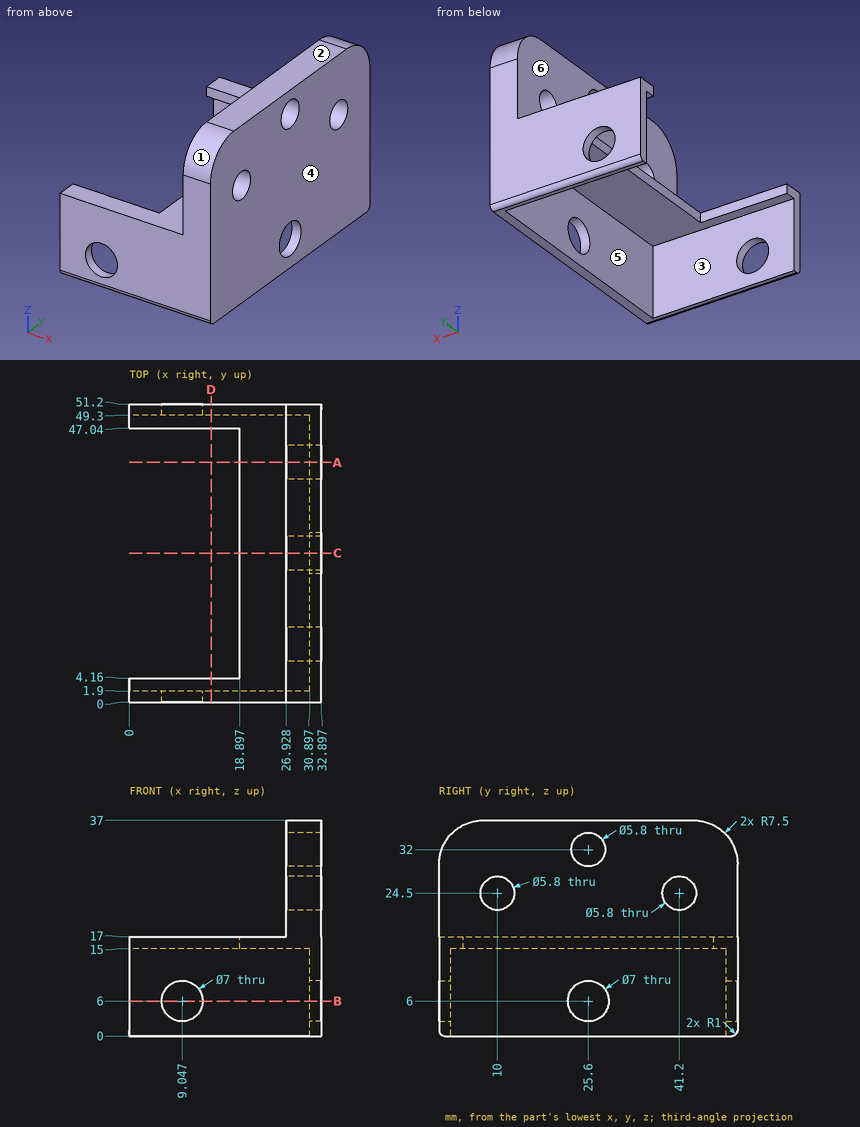
Answer from the drawing. Dimensions are ordinates in mm from the lowest x, y and z of the part. A direction names the side the tool comes from. Round coordinates to 2 decimals unless told otherwise and drop trailing zeros. Loops run counter-clockwise (first coordinate to the right, second up) from the corner with the lowest first, then second, coordinate; pieces in that order, holes last.
Q1. Determine the mould class of the marked faces 1, 2 and 3 for opening direction Y: released by +Y, released by -Y, zero draft, split by the parting line, or undercut.
Q2. Each of these flat-tipped pins is pushed along its axis until it touches: pin 1 (1.6 mm diameter, centred on y = 16, z = 16, fed in from -X); pin 2 (6 mm diameter, centred on x = 23.5, y = 45.5, fed in from -Z); pin 3 (12 mm diameter, centred on y = 35, z = 8.5, fed in from -X). Where does it stop, or does it pass through?
Q3. Section C-C on y = 25.6 is taken. Write down the section's boundary in (x, z).
Q4. Which of the six approach directions +Z, -Z, +X, -X, +Y, -Y give full straight-line access (tool end or side, diameter ignored) to the marked faces 4, 5 and 6?
Q5. Consider probe 1 along X at (y, z) = (50, 6); probe 2 along Y at (x, z) = (12.5, 12); probe 3 along Y at (x, z) = (27, 22.5). Determine where each line is inside the solid, lowest interval first.
Q6. Section B-B on z = 6 is taken. Write down the section's boundary in (x, y), and give its area (3 significant figures).
Q7. Section A-A on y = 41.2 is taken. Write down the section's boundary in (x, z).
Q8. Section D-D on x = 14 is taken. Write down the section's boundary in (y, z).
Output:
1. face 1: released by -Y
1. face 2: zero draft
1. face 3: undercut
2. pin 1: stops at x = 18.9
2. pin 2: stops at z = 15
2. pin 3: stops at x = 30.9
3. outline: (18.9, 15) - (30.9, 15) - (30.9, 9.5) - (32.9, 9.5) - (32.9, 29.1) - (26.93, 29.1) - (26.93, 17) - (18.9, 17) - close; (26.93, 34.9) - (32.9, 34.9) - (32.9, 37) - (26.93, 37) - close; (30.9, 0) - (32.9, 0) - (32.9, 2.5) - (30.9, 2.5) - close
4. face 4: +Z, -Z, +X, +Y, -Y
4. face 5: -Z, -X
4. face 6: +Z, -X, +Y, -Y
5. probe 1: x = 0 to 5.55, 12.55 to 32.9
5. probe 2: y = 0 to 1.9, 49.3 to 51.2
5. probe 3: y = 0 to 7.9, 12.1 to 39.1, 43.3 to 51.2
6. outline: (0, 0) - (5.55, 0) - (5.55, 1.9) - (0, 1.9) - close; (0, 49.3) - (5.55, 49.3) - (5.55, 51.2) - (0, 51.2) - close; (12.55, 0) - (32.9, 0) - (32.9, 22.1) - (30.9, 22.1) - (30.9, 1.9) - (12.55, 1.9) - close; (12.55, 49.3) - (30.9, 49.3) - (30.9, 29.1) - (32.9, 29.1) - (32.9, 51.2) - (12.55, 51.2) - close
6. area: 179 mm2
7. outline: (18.9, 15) - (30.9, 15) - (30.9, 0) - (32.9, 0) - (32.9, 21.6) - (26.93, 21.6) - (26.93, 17) - (18.9, 17) - close; (26.93, 27.4) - (32.9, 27.4) - (32.9, 37) - (26.93, 37) - close
8. outline: (0, 1) arc R1 ccw to (1, 0) - (1.9, 0) - (1.9, 15) - (4.16, 15) - (4.16, 17) - (0, 17) - close; (47.04, 15) - (49.3, 15) - (49.3, 0) - (50.2, 0) arc R1 ccw to (51.2, 1) - (51.2, 17) - (47.04, 17) - close
